Autodesk Fusion 360 part; units mm, degrees
sketch "Sketch1" plane through (0, 0, 0) normal (0, 0, 1) x (1, 0, 0)
  circle A0 centre (0, 0) radius 17
  line L0 (12, 58.7878) -> (12, 68.9638)
  line L1 (-12, 58.7878) -> (-12, 68.9638)
  arc A1 (12, 68.9638) -> (-12, 68.9638) centre (0, 0) ccw
  line L2 (-50.0545, 33.0839) -> (-57.25, 40.2795)
  arc A2 (-40.2795, 57.25) -> (-57.25, 40.2795) centre (0, 0) ccw
  line L3 (-33.0839, 50.0545) -> (-40.2795, 57.25)
  line L4 (-58.7878, -12) -> (-68.9638, -12)
  arc A3 (-68.9638, 12) -> (-68.9638, -12) centre (0, 0) ccw
  line L5 (-58.7878, 12) -> (-68.9638, 12)
  line L6 (-33.0839, -50.0545) -> (-40.2795, -57.25)
  arc A4 (-57.25, -40.2795) -> (-40.2795, -57.25) centre (0, 0) ccw
  line L7 (-50.0545, -33.0839) -> (-57.25, -40.2795)
  line L8 (12, -58.7878) -> (12, -68.9638)
  arc A5 (-12, -68.9638) -> (12, -68.9638) centre (0, 0) ccw
  line L9 (-12, -58.7878) -> (-12, -68.9638)
  line L10 (50.0545, -33.0839) -> (57.25, -40.2795)
  arc A6 (40.2795, -57.25) -> (57.25, -40.2795) centre (0, 0) ccw
  line L11 (33.0839, -50.0545) -> (40.2795, -57.25)
  line L12 (58.7878, 12) -> (68.9638, 12)
  arc A7 (68.9638, -12) -> (68.9638, 12) centre (0, 0) ccw
  line L13 (58.7878, -12) -> (68.9638, -12)
  line L14 (33.0839, 50.0545) -> (40.2795, 57.25)
  arc A8 (57.25, 40.2795) -> (40.2795, 57.25) centre (0, 0) ccw
  line L15 (50.0545, 33.0839) -> (57.25, 40.2795)
  line L16 (31.6697, 51.4687) -> (33.0839, 50.0545) construction
  line L17 (14, 58.7878) -> (12, 58.7878) construction
  arc A9 (12, 58.7878) -> (15.7853, 57.8863) centre (14, 58.7878) ccw
  arc A10 (29.7699, 52.0937) -> (33.0839, 50.0545) centre (31.6697, 51.4687) ccw
  arc A11 (29.7699, 52.0937) -> (15.7853, 57.8863) centre (0, 0) ccw
  arc A12 (-15.7853, 57.8863) -> (-29.7699, 52.0937) centre (0, 0) ccw
  arc A13 (-52.0937, 29.7699) -> (-57.8863, 15.7853) centre (0, 0) ccw
  arc A14 (15.7853, -57.8863) -> (29.7699, -52.0937) centre (0, 0) ccw
  arc A15 (-57.8863, -15.7853) -> (-52.0937, -29.7699) centre (0, 0) ccw
  arc A16 (-29.7699, -52.0937) -> (-15.7853, -57.8863) centre (0, 0) ccw
  arc A17 (52.0937, -29.7699) -> (57.8863, -15.7853) centre (0, 0) ccw
  arc A18 (57.8863, 15.7853) -> (52.0937, 29.7699) centre (0, 0) ccw
  arc A19 (-33.0839, 50.0545) -> (-29.7699, 52.0937) centre (-31.6697, 51.4687) ccw
  arc A20 (-15.7853, 57.8863) -> (-12, 58.7878) centre (-14, 58.7878) ccw
  arc A21 (-58.7878, 12) -> (-57.8863, 15.7853) centre (-58.7878, 14) ccw
  arc A22 (-52.0937, 29.7699) -> (-50.0545, 33.0839) centre (-51.4687, 31.6697) ccw
  arc A23 (-50.0545, -33.0839) -> (-52.0937, -29.7699) centre (-51.4687, -31.6697) ccw
  arc A24 (-57.8863, -15.7853) -> (-58.7878, -12) centre (-58.7878, -14) ccw
  arc A25 (-12, -58.7878) -> (-15.7853, -57.8863) centre (-14, -58.7878) ccw
  arc A26 (-29.7699, -52.0937) -> (-33.0839, -50.0545) centre (-31.6697, -51.4687) ccw
  arc A27 (33.0839, -50.0545) -> (29.7699, -52.0937) centre (31.6697, -51.4687) ccw
  arc A28 (15.7853, -57.8863) -> (12, -58.7878) centre (14, -58.7878) ccw
  arc A29 (58.7878, -12) -> (57.8863, -15.7853) centre (58.7878, -14) ccw
  arc A30 (52.0937, -29.7699) -> (50.0545, -33.0839) centre (51.4687, -31.6697) ccw
  arc A31 (50.0545, 33.0839) -> (52.0937, 29.7699) centre (51.4687, 31.6697) ccw
  arc A32 (57.8863, 15.7853) -> (58.7878, 12) centre (58.7878, 14) ccw
  dimension "d1" = 140
  dimension "d2" = 120
  dimension "d3" = 34
  dimension "d4" = 24
  dimension "d7" = 360
  dimension "d8" = 4
  dimension "d9" = 4
  dimension "d11" = 360
extrude "Extrude1" add sketch "Sketch1" along normal blind 46 and the other way blind 121 contours A0
extrude "Extrude2" add sketch "Sketch1" against normal blind 64
sketch "Sketch2" plane through (0, 0, -121) normal (0, 0, -1) x (1, 0, 0)
  circle A0 centre (0, 0) radius 17
  circle A1 centre (0, 0) radius 13
  dimension "d18" = 26
extrude "Extrude3" add sketch "Sketch2" along normal blind 42 contours A1
ref_plane "WorkPlane1" through (0, 17, 24.5322) normal (0, 1, 0) x (1, 0, 0)
ref_plane "WorkPlane2" through (0, -12.224, 24.5322) normal (0, 1, 0) x (1, 0, 0)
sketch "Sketch3" plane through (0, -12.224, 24.5322) normal (0, 1, 0) x (1, 0, 0)
  line L0 (0, -21) -> (0, 21) construction
  line L1 (-4.9514, 8.6954) -> (-4.9514, -21.5)
  line L2 (4.9987, 8.1155) -> (4.9987, -21.5)
  line L3 (4.9987, -21.5) -> (-4.9514, -21.5)
  arc A0 (4.9987, 7.8845) -> (-4.9514, 7.3046) centre (0, 8) ccw
  dimension "d23" = 10
  dimension "d24" = 29
extrude "Extrude4" cut sketch "Sketch3" against normal blind 13 contours L1 L2 L3 A0
ref_plane "WorkPlane3" through (0, -17, -95.604) normal (0, -1, 0) x (-1, 0, 0)
sketch "Sketch4" plane through (0, 0, 0) normal (0, 0, 1) x (1, 0, 0)
sketch "Sketch5" plane through (0, -17, -95.604) normal (0, -1, 0) x (1, 0, 0)
  line L0 (-4.9938, 15.8882) -> (-5, -18.8629)
  line L1 (4.9938, 15.8882) -> (5, -18.8629)
  arc A0 (-4.9514, 111.4408) -> (4.9987, 112.0207) centre (0, 112.1362) ccw
  arc A1 (4.9938, 15.8882) -> (-4.9938, 15.8882) centre (0, 16.1362) ccw
  arc A2 (-5, -18.8629) -> (5, -18.8629) centre (0, -18.8638) ccw
  dimension "d28" = 10
  dimension "d29" = 10
  dimension "d30" = 35
  dimension "d31" = 96
extrude "Extrude5" cut sketch "Sketch5" against normal blind 20
chamfer "Chamfer1" distance 2 angle 45 2 edges at (-12.1203, 4.701, -163) (-0.0247, 17, 46)
chamfer "Chamfer2" distance 1 angle 45 1 edges at (-15.8496, 6.1475, -121)
fillet "Fillet1" radius 4 1 edges at (-15.8496, 6.1475, -64)
Design review of the part built by this model. Coordinates are the model's own, in mm. A direction names the side the tool comes from. Round coordinates to 2 decimals unless told otherwise and drop trailing zeros. Write each loop counter-clockwise with the first axis right and the second up, starting at its lowest first coordinate (ties: lowest second). Pieces come first, ordered by that corner, then holes. Notation, with made-up numbers: (31.5, -16.5) -> (36.5, -16.5) arc R24 ccw to (36.5, 4.5) -> close; hole circle Ø7 at (54.5, 45.25). An arc over 180 degrees is marked (long way). Answer in a Markdown table with one row per item.
Q1. Draft analysis for pull direction X (two halves, no side actions). For faces 1 (the face through (-36.63, -53.6, -31.55)), 2 (the face through (15, 17, 0)), 3 (the face through (-55.473, -22.863, -31.552)), state which applies: +X half, -X half, draft (parallel to the pull), parting line (faces both ways), or undercut.
The answers:
| item | result |
|---|---|
| face 1 | undercut |
| face 2 | draft |
| face 3 | -X half |
Q2. For faces 4 (the face through (23.06, 55.39, -31.55)), 5 (the face through (-53.6, 36.63, -31.55)), 6 (the face through (12, -64, -32)), list the 3-axis set-ups (+Z, -Z, +X, -X, +Y, -Y) from which the entire face can be reached by the end or side of a thin tool; tool diameter is ignored.
The answers:
| item | result |
|---|---|
| face 4 | +Z, -Z, +Y |
| face 5 | +Z, -Z, -X |
| face 6 | +Z, -Z, +X, -Y |
Q3. Take a section at A-A, the plane y = 0. State the section outline as (x, z) points.
The answers:
| item | result |
|---|---|
| outline | (-70, -64) -> (-21, -64) arc R4 cw to (-17, -68) -> (-17, -120) -> (-16, -121) -> (-13, -121) -> (-13, -161) -> (-11, -163) -> (11, -163) -> (13, -161) -> (13, -121) -> (16, -121) -> (17, -120) -> (17, -68) arc R4 cw to (21, -64) -> (70, -64) -> (70, 0) -> (17, 0) -> (17, 44) -> (15, 46) -> (-15, 46) -> (-17, 44) -> (-17, 0) -> (-70, 0) -> close; hole (-5, -114.47) arc R5 ccw to (5, -114.47) -> (4.99, -79.72) arc R5 ccw (long way) to (-4.99, -79.72) -> close |
Q4. To check wall thickness, follow L1, parallel to Y at x = 51, z = -50; L2, parallel to Y at x = -0.5, z = -27; L3, parallel to Z at x = 25.5, y = 17. State the ranges of each line that lie inside material, in increasing order. Write a range as [from, to].
The answers:
| item | result |
|---|---|
| L1 | [-47.95, -34.03], [-29.73, 29.73], [34.03, 47.95] |
| L2 | [-70, 70] |
| L3 | [-64, 0] |
Q5. Take a section at C-C, the plane y = 45.5. State the section outline as (x, z) points.
The answers:
| item | result |
|---|---|
| outline | (-53.2, -64) -> (53.2, -64) -> (53.2, 0) -> (-53.2, 0) -> close |
Q6. Clearance check with flat-ended pins moving along their axes: pin 1 Ø1 at (y, z) = (-5.5, 2) entering from -X; pin 2 Ø6 at (x, z) = (-2.5, -74.5) entering from +Y; pin 3 Ø11 at (y, z) = (62, -43) entering from +X. State where each tip first meets the part, or that it passes through.
The answers:
| item | result |
|---|---|
| pin 1 | x = -16.25 |
| pin 2 | y = 17 |
| pin 3 | x = 41.32 |
